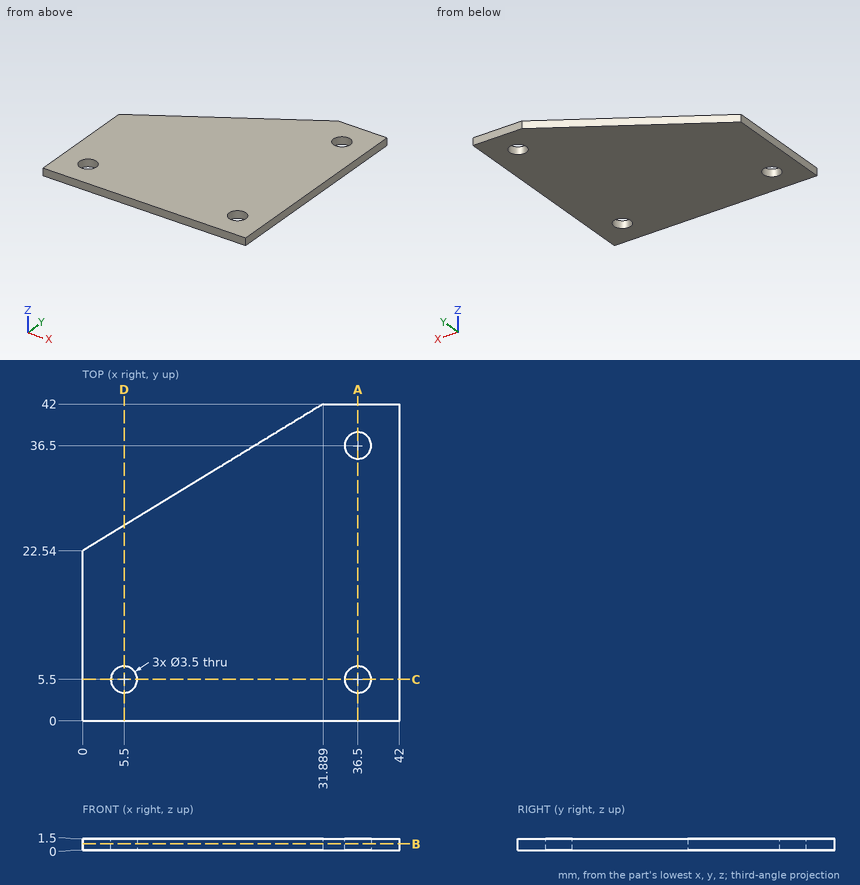
Geometry check sheet. Reference: drawing and pictorial views, mm from the part's lowest x, y, z. Round coordinates to 2 decimals unless told otherwise and drop trailing zeros. Loops run counter-clockwise (first coordinate to the right, second up) from the corner with the lowest first, then second, coordinate; pieces in that order, holes last. Notation, with made-up numbers: (33, -33) -> (59, -33) arc R34 ccw to (59, 3) -> close; hole circle Ø7 at (87.25, 84). An arc over 180 degrees is marked (long way). Answer as a JSON object with one key per item and string values. Group by question number.
Item 1: Cross-section at D-D, the plane x = 5.5. Record the cut outline in (y, z).
Item 2: Cross-section at B-B, the plane z = 0.85. Record the cut outline in (x, y).
Item 3: Thickness scan on line 1 along Y through (x, z) = (36.5, 0.4); line 2 along X through (y, z) = (6, 0.15); line 3 along X through (y, z) = (37, 1.1) (1 decimal). Record the ranges inside material, lowest first.
Item 4: Depth check by flat-ended pin: pin 1 Ø2 at (x, y) = (36.5, 5.5) entering from +Z. Enter the tip coordinate at first touch or a pass-through.
Item 5: Cross-section at A-A, the plane x = 36.5. Record the cut outline in (y, z).
Determined:
{
 "1": {"outline": "(0, 0) -> (3.75, 0) -> (3.75, 1.5) -> (0, 1.5) -> close; (7.25, 0) -> (25.9, 0) -> (25.9, 1.5) -> (7.25, 1.5) -> close"},
 "2": {"outline": "(0, 0) -> (42, 0) -> (42, 42) -> (31.89, 42) -> (0, 22.54) -> close; hole circle Ø3.5 at (5.5, 5.5); hole circle Ø3.5 at (36.5, 5.5); hole circle Ø3.5 at (36.5, 36.5)"},
 "3": {"line 1": "y = 0 to 3.75, 7.25 to 34.75, 38.25 to 42", "line 2": "x = 0 to 3.82, 7.18 to 34.82, 38.18 to 42", "line 3": "x = 23.7 to 34.8, 38.2 to 42"},
 "4": {"pin 1": "passes through"},
 "5": {"outline": "(0, 0) -> (3.75, 0) -> (3.75, 1.5) -> (0, 1.5) -> close; (7.25, 0) -> (34.75, 0) -> (34.75, 1.5) -> (7.25, 1.5) -> close; (38.25, 0) -> (42, 0) -> (42, 1.5) -> (38.25, 1.5) -> close"}
}
